```python
from build123d import *

# Parameters (mm, degrees)
DODANIE_WYCI_GNI_CIE1_DEPTH = 20
WYTNIJ_WYCI_GNI_CIE1_DEPTH  = 4
SZKIC2_W                    = 8
SZKIC2_H                    = 1
WYTNIJ_WYCI_GNI_CIE2_DEPTH  = 27.004807248
SZKIC2_3_R                  = 1.5
WYTNIJ_WYCI_GNI_CIE3_DEPTH  = 5.5
SZKIC2_4_R                  = 1.5
WYTNIJ_WYCI_GNI_CIE4_DEPTH  = 27.004807325
ZAOKR_GLENIE1_R             = 1
ZAOKR_GLENIE2_R             = 1
ZAOKR_GLENIE3_R             = 1
ZAOKR_GLENIE4_R             = 0.5
ZAOKR_GLENIE5_R             = 0.5


with BuildPart() as part:
    # Szkic1 → Dodanie-wyciągnięcie1 (new body)
    with BuildSketch(Plane(origin=(0, 0, 0), x_dir=(1, 0, 0), z_dir=(0, 1, 0))):
        with BuildLine():
            Line((9.2, 1.55), (12, 1.55))
            Line((12, 1.55), (12, 5.75))
            Line((12, 5.75), (-12, 5.75))
            Line((-12, 5.75), (-12, 0))
            Line((-12, 0), (-6.321637353, 0))
            ThreePointArc((-6.321637353, 0), (-4, 1.1), (-1.678362647, 0))
            Line((-1.678362647, 0), (0.772821971, 0))
            ThreePointArc((0.772821971, 0), (3.5, 1.75), (6.227178029, 0))
            Line((6.227178029, 0), (7.65, 0))
            ThreePointArc((7.65, 0), (8.103984489, 1.096015511), (9.2, 1.55))
        make_face()
        with BuildLine():
            Line((-6.321637353, 0), (-12, 0))
            Line((-12, 0), (-12, -1.15))
            Line((-12, -1.15), (-6.90473751, -1.15))
            ThreePointArc((-6.90473751, -1.15), (-6.675700572, -0.543303111), (-6.321637353, 0))
        make_face()
        with BuildLine():
            Line((12, -5.75), (12, -1.55))
            Line((12, -1.55), (9.2, -1.55))
            ThreePointArc((9.2, -1.55), (8.103984489, -1.096015511), (7.65, 0))
            Line((7.65, 0), (6.227178029, 0))
            ThreePointArc((6.227178029, 0), (6.431001031, -0.610286817), (6.5, -1.25))
            ThreePointArc((6.5, -1.25), (2.860286817, -4.181001031), (0.772821971, 0))
            Line((0.772821971, 0), (-1.678362647, 0))
            ThreePointArc((-1.678362647, 0), (-2.643303111, -4.575700572), (-6.90473751, -2.65))
            Line((-6.90473751, -2.65), (-12, -2.65))
            Line((-12, -2.65), (-12, -5.75))
            Line((-12, -5.75), (12, -5.75))
        make_face()
        with BuildLine():
            Line((12, -1.55), (12, 0))
            Line((12, 0), (10.75, 0))
            ThreePointArc((10.75, 0), (10.296015511, -1.096015511), (9.2, -1.55))
            Line((9.2, -1.55), (12, -1.55))
        make_face()
        with BuildLine():
            Line((10.75, 0), (12, 0))
            Line((12, 0), (12, 1.55))
            Line((12, 1.55), (9.2, 1.55))
            ThreePointArc((9.2, 1.55), (10.296015511, 1.096015511), (10.75, 0))
        make_face()
    extrude(amount=-DODANIE_WYCI_GNI_CIE1_DEPTH)

    # Szkic1<4> → Wytnij-wyciągnięcie1 (cut)
    with BuildSketch(Plane(origin=(0, 0, 0), x_dir=(1, 0, 0), z_dir=(0, 1, 0))):
        with BuildLine():
            Line((10.75, 0), (12, 0))
            Line((12, 0), (12, 1.55))
            Line((12, 1.55), (9.2, 1.55))
            ThreePointArc((9.2, 1.55), (10.296015511, 1.096015511), (10.75, 0))
        make_face()
        with BuildLine():
            Line((12, -1.55), (12, 0))
            Line((12, 0), (10.75, 0))
            ThreePointArc((10.75, 0), (10.296015511, -1.096015511), (9.2, -1.55))
            Line((9.2, -1.55), (12, -1.55))
        make_face()
    extrude(amount=-WYTNIJ_WYCI_GNI_CIE1_DEPTH, mode=Mode.SUBTRACT)

    # Szkic2 → Wytnij-wyciągnięcie2 (cut, through all)
    with BuildSketch(Plane.XY.offset(5.75)):
        with Locations((-8, -0.5)):
            Rectangle(SZKIC2_W, SZKIC2_H)
    extrude(amount=-WYTNIJ_WYCI_GNI_CIE2_DEPTH, mode=Mode.SUBTRACT)

    # Szkic2<3> → Wytnij-wyciągnięcie3 (cut)
    with BuildSketch(Plane.XY.offset(5.75)):
        with Locations((9.2, -10)):
            Circle(SZKIC2_3_R)
    extrude(amount=-WYTNIJ_WYCI_GNI_CIE3_DEPTH, mode=Mode.SUBTRACT)

    # Szkic2<4> → Wytnij-wyciągnięcie4 (cut, through all)
    with BuildSketch(Plane.XY.offset(5.75)):
        with Locations((-9.5, -5)):
            Circle(SZKIC2_4_R)
        with Locations((-9.5, -14.5)):
            Circle(SZKIC2_4_R)
    extrude(amount=-WYTNIJ_WYCI_GNI_CIE4_DEPTH, mode=Mode.SUBTRACT)

    # Zaokrąglenie1
    zaokr_glenie1_edges = [part.edges().sort_by_distance(p)[0] for p in [
        (-4, -1, -3.425),
        (-4, -1, 5.325),
    ]]
    fillet(zaokr_glenie1_edges, radius=ZAOKR_GLENIE1_R - 0.0001)  # a hair under: the kernel refuses the full size

    # Zaokrąglenie2
    zaokr_glenie2_edges = [part.edges().sort_by_distance(p)[0] for p in [
        (-4, 0, 5.325),
        (-4, 0, -3.425),
    ]]
    fillet(zaokr_glenie2_edges, radius=ZAOKR_GLENIE2_R)

    # Zaokrąglenie3
    zaokr_glenie3_edges = [part.edges().sort_by_distance(p)[0] for p in [
        (12, -2, -1.55),
        (12, -2, 1.55),
    ]]
    fillet(zaokr_glenie3_edges, radius=ZAOKR_GLENIE3_R)

    # Zaokrąglenie4
    zaokr_glenie4_edges = [part.edges().sort_by_distance(p)[0] for p in [
        (-4.499937501, -0.866031585, -5.75),
        (-4.499937501, -0.866031585, 5.75),
        (-3.767919429, -0.133981813, 5.75),
        (-3.767919429, -0.133981813, -5.75),
        (12, 0, -4.15),
        (11.707106781, 0, -1.842893219),
        (11.707106781, 0, 1.842893219),
        (4.366046536, 0, -5.75),
        (12, 0, 4.15),
        (4.366046536, 0, 5.75),
        (0, -20, 5.75),
        (-12, -10.5, 5.75),
        (-12, -10.5, -5.75),
        (12, -10, -5.75),
        (12, -10, 5.75),
        (0, -20, -5.75),
        (-12, -20, -2.3),
        (7.65, 0, 0),
        (10.1, 0, -1.55),
        (10.1, 0, 1.55),
        (-12, -20, 4.2),
        (-8.49995, -1, -5.75),
        (-12, -1, 4.2),
        (-12, -1, -2.3),
        (-8.49995, -1, 5.75),
    ]]
    fillet(zaokr_glenie4_edges, radius=ZAOKR_GLENIE4_R)

    # Zaokrąglenie5
    zaokr_glenie5_edges = [part.edges().sort_by_distance(p)[0] for p in [
        (12, -4, 0),
    ]]
    fillet(zaokr_glenie5_edges, radius=ZAOKR_GLENIE5_R)


solid = part.part
```
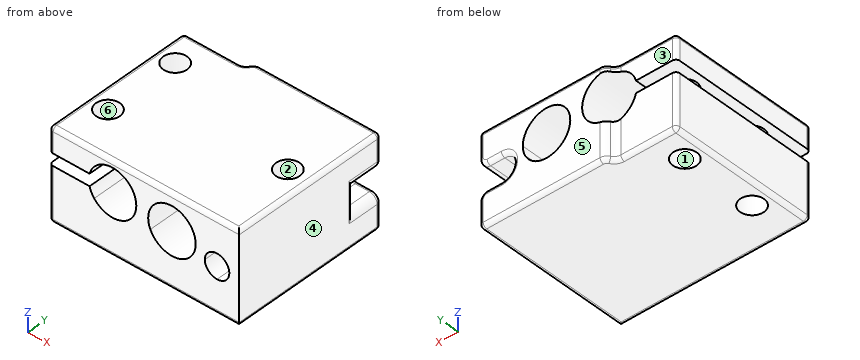
Verification items for the finished model (mm, model axes). Face numbers are marked on the shaded views. A direction names the side the tool comes from. Round coordinates to 2 decimals unless told otherwise and drop trailing zeros. Order: outer loops, then holes, each group sorted by start corner. A loop starts at its lowest first (then second) coordinate and runs counter-clockwise, first axis right, second up. Notation, with made-up numbers: (-39, 53.25) -> (-14, 53.25) arc R25 ccw to (-14, 74.25) -> close; hole circle Ø9 at (30.5, 54). An arc over 180 degrees is marked (long way). Put each result on its own line as item: value. Start each with the question number.
(1) Draft check along X on the marked faces 4, 5 and 6. Enter one of: +X half, -X half, draft (parallel to the pull), parting line (faces both ways), or undercut.
(2) Depth check by flat-ended pin: pin 1 Ø1.8 at (x, y) = (-9.5, -5) entering from +Z; pin 2 Ø2 at (x, z) = (-9.5, 4.5) entering from +Y; pin 3 Ø0.7 at (x, z) = (10.5, 0) entering from +Y. Enter the tip coordinate at first touch or a pass-through.
(3) Section check A-A (y = -14.5). Enter the section's corners in (x, z), then the cut area to 3 significant figures.
(4) Tool access check on the marked faces 1, 2 and 3. Record the directions out of +Z, -Z, +X, -X, +Y, -Y that give a thin tool (end or side, any length) a straight path to the whole face; none if there is none.
(5) Section check C-C (x = 3.5). Enter the section's corners in (y, z).
(6) Section check D-D (x = 9.5). State how many separate pieces and enclosed holes the cut face has, then the cut area to 3 significant figures.
(7) Section check B-B (y = -7.25). Enter the section's corners in (x, z), then the cut area to 3 significant figures.
(8) Material ranges on line 1 along X through (y, z) = (-17.75, 0); line 2 along Y through (x, z) = (-9.5, -2.25); line 3 along X through (y, z) = (-11, 1.25), recorded low to high.
Completed:
1. face 4: +X half
1. face 5: draft
1. face 6: undercut
2. pin 1: passes through
2. pin 2: stops at y = -1
2. pin 3: stops at y = -4
3. outline: (-12, -5.25) arc R0.5 ccw to (-11.5, -5.75) -> (-11, -5.75) -> (-11, 1.15) -> (-12, 1.15) -> close; (-12, 2.65) -> (-11, 2.65) -> (-11, 5.75) -> (-11.5, 5.75) arc R0.5 ccw to (-12, 5.25) -> close; (-8, -5.75) -> (11.5, -5.75) arc R0.5 ccw to (12, -5.25) -> (12, 5.25) arc R0.5 ccw to (11.5, 5.75) -> (-8, 5.75) -> (-8, 2.65) -> (-6.9, 2.65) arc R3 cw (long way) to (-6.9, 1.15) -> (-8, 1.15) -> close; hole circle Ø6 at (3.5, 1.25); hole circle Ø3.1 at (9.2, 0)
3. area: 174 mm2
4. face 1: +Z, -Z
4. face 2: +Z
4. face 3: +Z, -Z, -X, +Y
5. outline: (-20, -5.25) arc R0.5 ccw to (-19.5, -5.75) -> (-0.5, -5.75) arc R0.5 ccw to (0, -5.25) -> (0, -1.75) -> (-20, -1.75) -> close; (-20, 4.25) -> (0, 4.25) -> (0, 5.25) arc R0.5 ccw to (-0.5, 5.75) -> (-19.5, 5.75) arc R0.5 ccw to (-20, 5.25) -> close
6. separate pieces: 3
6. enclosed holes: 0
6. area: 156 mm2
7. outline: (-12, -5.25) arc R0.5 ccw to (-11.5, -5.75) -> (11.5, -5.75) arc R0.5 ccw to (12, -5.25) -> (12, 5.25) arc R0.5 ccw to (11.5, 5.75) -> (-11.5, 5.75) arc R0.5 ccw to (-12, 5.25) -> (-12, 2.65) -> (-6.9, 2.65) arc R3 cw (long way) to (-6.9, 1.15) -> (-12, 1.15) -> close; hole circle Ø6 at (3.5, 1.25); hole circle Ø3.1 at (9.2, 0)
7. area: 204 mm2
8. line 1: x = -12 to -6.32, -1.68 to 0.77, 6.23 to 7.65, 10.75 to 12
8. line 2: y = -20 to -16, -13 to -6.5, -3.5 to -1
8. line 3: x = -1.07 to 0.5, 6.5 to 8.08, 10.32 to 12
